from build123d import *

# Parameters (mm, degrees)
EXTRUDE_1_DEPTH = 4.8


with BuildPart() as part:
    # 草圖1 → 填料-伸長1 (new body)
    with BuildSketch(Plane(origin=(0, 0, 0), x_dir=(1, 0, 0), z_dir=(0, 1, 0))):
        with BuildLine():
            Line((-7, 1), (7, 1))
            Line((7, 1), (7, 3.3))
            Line((7, 3.3), (5.5, 3.3))
            Line((5.5, 3.3), (7.431056476, 7.371095386))
            ThreePointArc((7.431056476, 7.371095386), (7.665760023, 7.614923881), (8, 7.668043813))
            Line((8, 7.668043813), (8, 1))
            Line((8, 1), (8, 0))
            Line((8, 0), (-8, 0))
            Line((-8, 0), (-8, 1))
            Line((-8, 1), (-8, 7.668043813))
            ThreePointArc((-8, 7.668043813), (-7.665760023, 7.614923881), (-7.431056476, 7.371095386))
            Line((-7.431056476, 7.371095386), (-5.5, 3.3))
            Line((-5.5, 3.3), (-7, 3.3))
            Line((-7, 3.3), (-7, 1))
        make_face()
    extrude(amount=EXTRUDE_1_DEPTH)


solid = part.part
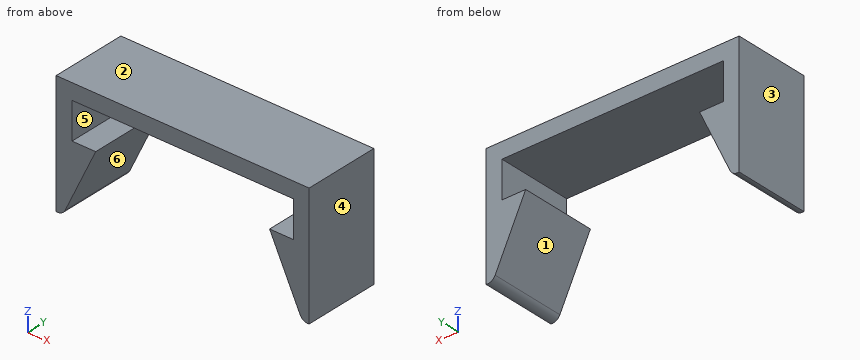
Here's how the part is built. I have some questions about the finished solid (model axes, mm). Face numbers are marked on the shaded views. A direction names the side the tool comes from. Give positions to 0.01 mm unless a question says otherwise; leave off trailing zeros. Loops run counter-clockwise (first coordinate to the right, second up) from the corner with the lowest first, then second, coordinate; pieces in that order, holes last. Notation, with made-up numbers: (6, 4) -> (62, 4) arc R15 ccw to (62, 10) -> close; hole circle Ø3 at (88.25, 31.5). An arc over 180 degrees is marked (long way). Answer as a JSON object with one key per item and string values. Group by question number.
Item 1: I need wall thicknesses on L1, parallel to X at y = 4.3, z = -1.5; L2, parallel to Z at x = 4.5, y = 1.85; L3, parallel to Z at x = 6.75, y = 4.25. Which ranges of each line are inside material? Lowest first, please.
Item 2: Imagine slicing it at A-A on z = -3. Write out the boundary of the cut face in (x, y).
Item 3: Imagine slicing it at C-C on y = 4.4. Write out the boundary of the cut face in (x, z), then the cut area to 3 significant figures.
Item 4: Imagine slicing it at B-B on x = -6. Write out the boundary of the cut face in (y, z), then the cut area to 3 significant figures.
Item 5: Thinking about a two-plate mould opening in X: for the marked faces 1, 2 and 3, which applies, pulls with the +X half, pulls with the -X half, needs draft (parallel to the pull), parting line crosses it, or undercut?
Item 6: Imagine slicing it at D-D on x = -2.25. Write out the boundary of the cut face in (y, z), then the cut area to 3 significant figures.
Item 7: On a 3-axis mill with a long thin cutter (end or side, diameter ignored), from which of +Z, -Z, +X, -X, +Y, -Y can I reach the whole of each face in a straight line? I mean the marked faces 4, 5 and 6. Say none if no direction works.
Answer list:
{
 "1": {"L1": "x = -8 to -7, 7 to 8", "L2": "z = -1 to 0", "L3": "z = -5.94 to -3.3, -1 to 0"},
 "2": {"outline": "(-8, 0) -> (-7, 0) -> (-7, 4.8) -> (-8, 4.8) -> close; (7, 0) -> (8, 0) -> (8, 4.8) -> (7, 4.8) -> close"},
 "3": {"outline": "(-8, -7.67) arc R0.53 ccw to (-7.43, -7.37) -> (-5.5, -3.3) -> (-7, -3.3) -> (-7, -1) -> (7, -1) -> (7, -3.3) -> (5.5, -3.3) -> (7.43, -7.37) arc R0.53 ccw to (8, -7.67) -> (8, 0) -> (-8, 0) -> close", "area": "33.4 mm2"},
 "4": {"outline": "(0, -4.35) -> (4.8, -4.35) -> (4.8, -3.3) -> (0, -3.3) -> close; (0, -1) -> (4.8, -1) -> (4.8, 0) -> (0, 0) -> close", "area": "9.86 mm2"},
 "5": {"face 1": "undercut", "face 2": "needs draft", "face 3": "pulls with the -X half"},
 "6": {"outline": "(0, -1) -> (4.8, -1) -> (4.8, 0) -> (0, 0) -> close", "area": "4.80 mm2"},
 "7": {"face 4": "+Z, -Z, +X, +Y, -Y", "face 5": "+Y, -Y", "face 6": "-Z, +Y, -Y"}
}
